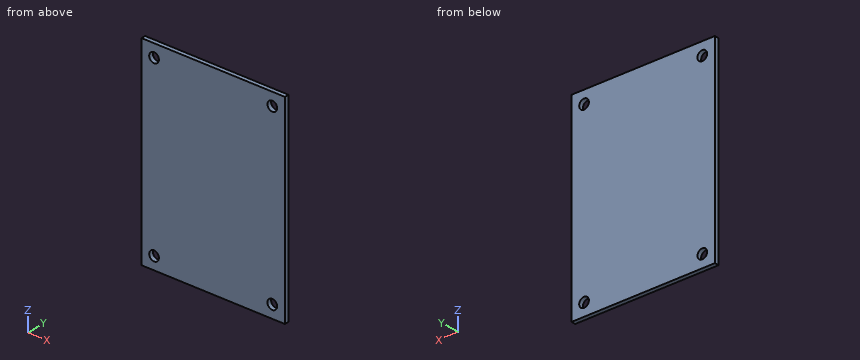
Autodesk Inventor part; units mm, degrees
ref_plane "YZ Plane" through (0, 0, 0) normal (1, 0, 0) x (0, 1, 0)
ref_plane "XZ Plane" through (0, 0, 0) normal (0, 1, 0) x (-1, 0, 0)
ref_plane "XY Plane" through (0, 0, 0) normal (0, 0, 1) x (1, 0, 0)
sketch "Sketch1" plane through (0, 0, 0) normal (0, 1, 0) x (-1, 0, 0)
  line L0 (20, 27.5) -> (-20, 27.5)
  line L1 (-20, 27.5) -> (-20, -27.5)
  line L2 (-20, -27.5) -> (20, -27.5)
  line L3 (20, -27.5) -> (20, 27.5)
  point P0 (0, 0)
  point P1 (20, 0)
  point P2 (0, -27.5)
  dimension "d0" = 55
  dimension "d1" = 40
extrude "Extrusion1" add sketch "Sketch1" along normal blind 1.2
sketch "Sketch2" plane through (0, 1.2, 0) normal (0, 1, 0) x (1, 0, 0)
  line L0 (-20, 27.5) -> (-20, -27.5)
  line L1 (20, -27.5) -> (20, 27.5)
  line L2 (-20, -27.5) -> (20, -27.5)
  line L3 (20, 27.5) -> (-20, 27.5)
  point P0 (0, 0)
  point P1 (-16.5, -24)
  point P2 (-16.5, 24)
  point P3 (16.5, -24)
  point P4 (16.5, 24)
  dimension "d4" = 3.5
  dimension "d5" = 3.5
  dimension "d6" = 3.5
  dimension "d7" = 3.5
hole "Hole1" at (-16.5, 1.2, 24) at (-16.5, 1.2, -24) at (16.5, 1.2, 24) at (16.5, 1.2, -24) direction (0, -1, 0) diameter 2.7 end through all
properties part number "rpcomputemodule4"
Geometry: final body of the model. Coordinates: model frame, mm. Give positions to 0.01 mm unless a question says otherwise; leave off trailing zeros. Write each loop counter-clockwise with the first axis right and the second up, starting at its lowest first coordinate (ties: lowest second). Pieces come first, ordered by that corner, then holes. Notation, with made-up numbers: M 60.25,-25 L 113.25,-25 A29 cw 113.25,-3 Z; hole C 32.5,6.25 d7. An arc over 180 degrees is marked long. Answer in a Markdown table with one row per item. Add a question column.
(1) Ray query, line 1 (Z direction, x = 16.5, y = 0.5); line 2 (X direction, y = 0.6, z = 24). Return the intervals inside material, ascending.
(2) Section B-B on x = 16.5. Return loops of the section in (y, z), and give its area (3 significant figures).
(3) Section A-A on z = -24. Return loops of the section in (x, y), and give its area (3 significant figures).
(4) First-contact query: pin 1 (1.6 mm diameter, centred on x = -16.5, z = -24, fed in from +Y). Flat tip, straight axial feed; report the tip coordinate or a pass-through.
Result set:
| question | item | result |
|---|---|---|
| 1 | line 1 | z = -27.5 to -25.35, -22.65 to 22.65, 25.35 to 27.5 |
| 1 | line 2 | x = -20 to -17.85, -15.15 to 15.15, 17.85 to 20 |
| 2 | outline | M 0,-27.5 L 1.2,-27.5 L 1.2,-25.35 L 0,-25.35 Z; M 0,-22.65 L 1.2,-22.65 L 1.2,22.65 L 0,22.65 Z; M 0,25.35 L 1.2,25.35 L 1.2,27.5 L 0,27.5 Z |
| 2 | area | 59.5 mm^2 |
| 3 | outline | M -20,0 L -17.85,0 L -17.85,1.2 L -20,1.2 Z; M -15.15,0 L 15.15,0 L 15.15,1.2 L -15.15,1.2 Z; M 17.85,0 L 20,0 L 20,1.2 L 17.85,1.2 Z |
| 3 | area | 41.5 mm^2 |
| 4 | pin 1 | passes through |
